from build123d import *

# Parameters (mm, degrees)
SKETCH1_W           = 25.4
SKETCH1_H           = 12.7
SKETCH1_R           = 5.08
SKETCH1_W_2         = 52.07
SKETCH1_H_2         = 6.35
SKETCH1_R_2         = 1.5875
BOSS_EXTRUDE1_DEPTH = 6.35
FILLET1_R           = 6.35
FILLET2_R           = 3.175


# Some blends are built 0.0001 mm under size
with BuildPart() as part:
    # Sketch1 → Boss-Extrude1 (new body)
    # profile 1 of 2: a face of its own
    with BuildSketch(Plane(origin=(0, 0, 0), x_dir=(1, 0, 0), z_dir=(0, 1, 0))):
        with Locations((12.7, 6.35)):
            Rectangle(SKETCH1_W, SKETCH1_H)
        with Locations(Location((19.05, 6.35, 0), (0, 0, 270))):
            Circle(SKETCH1_R, mode=Mode.SUBTRACT)
        with Locations(Location((6.35, 6.35, 0), (0, 0, 270))):
            Circle(SKETCH1_R, mode=Mode.SUBTRACT)
    # profile 2 of 2: a face of its own
    with BuildSketch(Plane(origin=(0, 0, 0), x_dir=(1, 0, 0), z_dir=(0, 1, 0))):
        with Locations((51.435, 6.35)):
            Rectangle(SKETCH1_W_2, SKETCH1_H_2)
        with Locations(Location((27.94, 6.35, 0), (0, 0, 270))):
            Circle(SKETCH1_R_2, mode=Mode.SUBTRACT)
        with Locations(Location((33.02, 6.35, 0), (0, 0, 270))):
            Circle(SKETCH1_R_2, mode=Mode.SUBTRACT)
        with Locations(Location((38.1, 6.35, 0), (0, 0, 270))):
            Circle(SKETCH1_R_2, mode=Mode.SUBTRACT)
        with Locations(Location((43.18, 6.35, 0), (0, 0, 270))):
            Circle(SKETCH1_R_2, mode=Mode.SUBTRACT)
        with Locations(Location((48.26, 6.35, 0), (0, 0, 270))):
            Circle(SKETCH1_R_2, mode=Mode.SUBTRACT)
        with Locations(Location((53.34, 6.35, 0), (0, 0, 270))):
            Circle(SKETCH1_R_2, mode=Mode.SUBTRACT)
        with Locations(Location((58.42, 6.35, 0), (0, 0, 270))):
            Circle(SKETCH1_R_2, mode=Mode.SUBTRACT)
        with Locations(Location((63.5, 6.35, 0), (0, 0, 270))):
            Circle(SKETCH1_R_2, mode=Mode.SUBTRACT)
        with Locations(Location((68.58, 6.35, 0), (0, 0, 270))):
            Circle(SKETCH1_R_2, mode=Mode.SUBTRACT)
        with Locations(Location((73.66, 6.35, 0), (0, 0, 270))):
            Circle(SKETCH1_R_2, mode=Mode.SUBTRACT)
    extrude(amount=BOSS_EXTRUDE1_DEPTH)

    # Fillet1
    # the kernel refuses this fillet: 6.35 mm, written as the material it takes off along each edge
    with BuildSketch(Plane(origin=(25.4, -13.748153285, -12.7), x_dir=(-1, 0, 0), z_dir=(0, 1, 0))) as fillet1_piece_1:
        with BuildLine():
            CenterArc((5.499261314, 6.35), FILLET1_R, 210, 60)
            Line((0, 3.175), (-0.109985226, 3.1115))
            ThreePointArc((-0.109985226, 3.1115), (-0.127, 1.5875), (-0.127, 0))
            Line((-0.127, 0), (0, -0.127))
            Line((0, -0.127), (5.499261314, -0.127))
            Line((5.499261314, -0.127), (5.499261314, 0))
        make_face()
    extrude(amount=33.84630657, mode=Mode.SUBTRACT)
    with BuildSketch(Plane(origin=(25.4, -13.748153285, 0), x_dir=(-1, 0, 0), z_dir=(0, 1, 0))) as fillet1_piece_2:
        with BuildLine():
            CenterArc((5.499261314, -6.35), FILLET1_R, 90, 60)
            Line((0, -3.175), (-0.109985226, -3.1115))
            ThreePointArc((-0.109985226, -3.1115), (-0.127, -1.5875), (-0.127, 0))
            Line((-0.127, 0), (0, 0.127))
            Line((0, 0.127), (5.499261314, 0.127))
            Line((5.499261314, 0.127), (5.499261314, 0))
        make_face()
    extrude(amount=33.84630657, mode=Mode.SUBTRACT)
    with BuildSketch(Plane(origin=(0, -15.875, -12.7), x_dir=(0, 0, 1), z_dir=(0, 1, 0)), Plane(origin=(0, -15.875, 0), x_dir=(1, 0, 0), z_dir=(0, 1, 0))) as fillet1_piece_3:
        with BuildLine():
            CenterArc((FILLET1_R, FILLET1_R), FILLET1_R, 180, 90)
            Line((0, FILLET1_R), (-FILLET1_R * 0.02, FILLET1_R))
            Line((-FILLET1_R * 0.02, FILLET1_R), (-FILLET1_R * 0.02, -FILLET1_R * 0.02))
            Line((-FILLET1_R * 0.02, -FILLET1_R * 0.02), (FILLET1_R, -FILLET1_R * 0.02))
            Line((FILLET1_R, -FILLET1_R * 0.02), (FILLET1_R, 0))
        make_face()
    extrude(amount=38.1, mode=Mode.SUBTRACT)

    # Fillet2
    fillet2_edges = [part.edges().sort_by_distance(p)[0] for p in [
        (77.47, 3.175, -9.525),
        (77.47, 3.175, -3.175),
    ]]
    fillet(fillet2_edges, radius=FILLET2_R - 0.0001)  # a hair under: the kernel refuses the full size


solid = part.part
Read the model definition and answer for the solid it produces. Units are mm, in the model's axes. A direction names the side the tool comes from. Coordinates: 2 decimals unless noted, no trailing zeros. Order: outer loops, then holes, each group sorted by start corner. A loop starts at its lowest first (then second) coordinate and runs counter-clockwise, first axis right, second up. Notation, with made-up numbers: (52.25, 65.5) -> (86.25, 65.5) arc R26 ccw to (86.25, 92.5) -> close; hole circle Ø11 at (12, 2.25). An arc over 180 degrees is marked (long way). Answer as a JSON object with one key per item and string values.
1) A cutting plane is placed at B-B, the plane y = 4.5. State how many separate pieces and enclosed holes the cut face has, plus the area to 3 significant figures.
Model answer:
{"separate pieces": "1", "enclosed holes": "12", "area": "380 mm²"}
2) Each of these flat-tipped pins is pushed along its axis until it touches: pin 1 (1 mm diameter, centred on x = 14, y = 2.5, fed in from +Z); pin 2 (3 mm diameter, centred on x = 47, y = 4.5, fed in from +Z) (3 decimals); pin 3 (3 mm diameter, centred on x = 68.58, z = -6.35, fed in from +Y) (3 decimals); pin 4 (2 mm diameter, centred on x = 54.5, y = 4, fed in from -Z) (3 decimals). Where does it stop, or does it pass through?
Model answer:
{"pin 1": "stops at z = 0", "pin 2": "stops at z = -3.175", "pin 3": "passes through", "pin 4": "stops at z = -9.525"}
3) A tool of negligible diameter and unlimited length cuts with its end or side. For faces 1 (the face through (0, 3.1, -6.5)), 2 (the face through (50, 3, -3.175)), from which of +Z, -Z, +X, -X, +Y, -Y can it reach the whole face along a straight path? Write none if from no direction.
Model answer:
{"face 1": "-X, +Y, -Y", "face 2": "+Z, +X, +Y, -Y"}
4) Consider line 1 along Z through (x, y) = (68.58, 2.75) (1 decimal); line 2 along X through (y, z) = (5, -10); line 3 along X through (y, z) = (2.75, -2.5). Determine where each line is inside the solid, lowest interval first. Write a range as from..to.
Model answer:
{"line 1": "z = -9.5..-7.9, -4.8..-3.2", "line 2": "x = 1.15..2.82, 9.88..15.52, 22.58..25.1", "line 3": "x = 1.3..3.04, 9.66..15.74, 22.36..24.95"}
5) A cutting plane is placed at A-A, the plane x = 19.05. Determine the outline of the cut face in (y, z).
Model answer:
{"outline": "(0, -12.7) -> (6.35, -12.7) -> (6.35, -11.43) -> (0, -11.43) -> close; (0, -1.27) -> (6.35, -1.27) -> (6.35, 0) -> (0, 0) -> close"}
6) The mould has two halves that part along X. Classify faces 3 (the face through (32.412, 3.131, -4.884)), 4 (the face through (50, 3, -9.525)), 5 (the face through (23.04, 3.13, -0.83)), 6 (the face through (65.074, 3.131, -6.557)): released by +X, released by -X, zero draft, split by the parting line, or undercut.
Model answer:
{"face 3": "undercut", "face 4": "zero draft", "face 5": "released by +X", "face 6": "undercut"}
